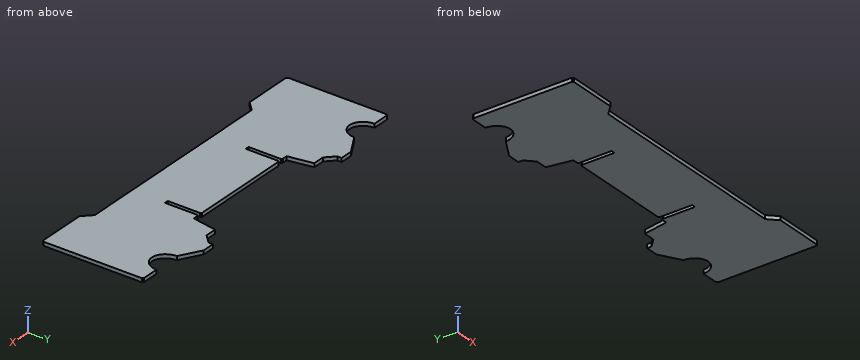
```python
from build123d import *

# Parameters (mm, degrees)
BOSS_EXTRUDE1_DEPTH = 3
SKETCH2_W           = 3
SKETCH2_H           = 4.791544689
CUT_EXTRUDE1_DEPTH  = 15
CHAMFER1_SIZE       = 1
CHAMFER2_SIZE       = 1


with BuildPart() as part:
    # Sketch1 → Boss-Extrude1 (new body)
    with BuildSketch(Plane.XY):
        with BuildLine():
            Line((93.184787819, -119.514382091), (261.489822447, -119.514382091))
            Line((261.489822447, -119.514382091), (268.560890259, -126.585449903))
            Line((268.560890259, -126.585449903), (308.560890259, -126.585449903))
            Line((308.560890259, -126.585449903), (308.560890259, -45.93363109))
            Line((308.560890259, -45.93363109), (294.267338786, -45.93363109))
            add(Edge.make_bspline(
                [(272.407878144, -45.934404782), (272.465337406, -47.438364471), (273.073186229, -50.465203155), (275.397677042, -54.367125899), (278.960411882, -57.115608226), (283.338040094, -58.12903526), (287.715596557, -57.115298346), (291.278136829, -54.366563828), (293.602351427, -50.464476548), (294.209985986, -47.437594843), (294.267338786, -45.93363109)],
                knots=[-1.525660034, -1.525660034, -1.525660034, -1.525660034, -1.144245025, -0.762830017, -0.381415008, 0, 0.381415008, 0.762830017, 1.144245025, 1.525660034, 1.525660034, 1.525660034, 1.525660034], degree=3))
            Line((272.407878144, -45.934404782), (256.337305133, -36.585449903))
            Line((256.337305133, -36.585449903), (246.337305133, -36.585449903))
            Line((246.337305133, -36.585449903), (246.337305133, -39.999663466))
            Line((246.337305133, -39.999663466), (239.751518696, -46.585449903))
            Line((239.751518696, -46.585449903), (230.574035326, -46.585449903))
            Line((230.574035326, -46.585449903), (227.127859803, -66.129682494))
            Line((227.127859803, -66.129682494), (127.546750463, -66.129682494))
            Line((127.546750463, -66.129682494), (124.10057494, -46.585449903))
            Line((124.10057494, -46.585449903), (114.923091571, -46.585449903))
            Line((114.923091571, -46.585449903), (108.337305133, -39.999663466))
            Line((108.337305133, -39.999663466), (108.337305133, -36.585449903))
            Line((108.337305133, -36.585449903), (98.337305133, -36.585449903))
            Line((98.337305133, -36.585449903), (82.267030577, -45.934761617))
            add(Edge.make_bspline(
                [(60.407579689, -45.934761617), (60.464998848, -47.438718586), (61.072758356, -50.465565598), (63.397111959, -54.367547882), (66.959733327, -57.116142381), (71.337305133, -58.129720884), (75.714876939, -57.116142381), (79.277498308, -54.367547882), (81.60185191, -50.465565598), (82.209611419, -47.438718586), (82.267030577, -45.934761617)],
                knots=[1.615943427, 1.615943427, 1.615943427, 1.615943427, 1.997355734, 2.37876804, 2.760180347, 3.141592654, 3.52300496, 3.904417267, 4.285829573, 4.66724188, 4.66724188, 4.66724188, 4.66724188], degree=3))
            Line((60.407579689, -45.934761617), (46.113720007, -45.934761617))
            Line((46.113720007, -45.934761617), (46.113720007, -126.585449903))
            Line((46.113720007, -126.585449903), (86.113720007, -126.585449903))
            Line((86.113720007, -126.585449903), (93.184787819, -119.514382091))
        make_face()
    extrude(amount=BOSS_EXTRUDE1_DEPTH)

    # Sketch2 → Cut-Extrude1 (cut)
    with BuildSketch(Plane(origin=(0, 0, 0), x_dir=(-1, 0, 0), z_dir=(0, 0, -1))):
        Polygon((-222.127859803, -66.129682494), (-222.127859803, -71.338137805), (-222.127859803, -92.822032293), (-219.127859803, -92.822032293), (-219.127859803, -71.338137805), (-219.127859803, -66.129682494), align=None)
        with Locations((-220.627859803, -63.73391015)):
            Rectangle(SKETCH2_W, SKETCH2_H)
        with Locations((-134.046750463, -63.73391015)):
            Rectangle(SKETCH2_W, SKETCH2_H)
        Polygon((-132.546750463, -66.129682494), (-135.546750463, -66.129682494), (-135.546750463, -71.338137805), (-135.546750463, -92.822032293), (-132.546750463, -92.822032293), (-132.546750463, -71.338137805), align=None)
    extrude(amount=-CUT_EXTRUDE1_DEPTH, mode=Mode.SUBTRACT)

    # Chamfer1
    chamfer1_edges = [part.edges().sort_by_distance(p)[0] for p in [
        (222.127859803, -66.129682494, 1.5),
        (219.127859803, -66.129682494, 1.5),
        (132.546750463, -66.129682494, 1.5),
        (135.546750463, -66.129682494, 1.5),
    ]]
    chamfer(chamfer1_edges, length=CHAMFER1_SIZE)

    # Chamfer2
    chamfer2_edges = [part.edges().sort_by_distance(p)[0] for p in [
        (308.560890259, -45.93363109, 1.5),
        (308.560890259, -126.585449903, 1.5),
        (46.113720007, -126.585449903, 1.5),
        (46.113720007, -45.934761617, 1.5),
    ]]
    chamfer(chamfer2_edges, length=CHAMFER2_SIZE)


solid = part.part
```
The model under review builds one solid part; all positions refer to its coordinate system, in mm. Round coordinates to 2 decimals unless told otherwise and drop trailing zeros. Write each loop counter-clockwise with the first axis right and the second up, starting at its lowest first coordinate (ties: lowest second). Pieces come first, ordered by that corner, then holes.
(1) Insertion check: pin 1 (1.5 mm diameter, centred on x = 201, z = 1.5, fed in from +Y); pin 2 (0.9 mm diameter, centred on x = 204.5, z = 1.5, fed in from -Y); pin 3 (1.5 mm diameter, centred on x = 117.5, z = 2, fed in from +Y). Each pin has a flat end and moves straight along its axis. Give the tip position at first contact, or say it passes through.
(2) We need section A-A on y = -85. Give the boundary of the cut face in (x, z), and give its area (3 significant figures).
(3) Wall thickness on L1, parallel to X at y = -88, z = 1.3; L2, parallel to X at y = -53.5, z = 2.05; L3, parallel to Y at x = 194, z = 0.75: over which ranges is each line inside the solid? List them lowest first.
(4) We need section B-B on x = 203.5. Give the boundary of the cut face in (y, z), and give its area (3 significant figures).
Findings below:
1. pin 1: stops at y = -66.13
1. pin 2: stops at y = -119.51
1. pin 3: stops at y = -46.59
2. outline: (46.11, 0) - (132.55, 0) - (132.55, 3) - (46.11, 3) - close; (135.55, 0) - (219.13, 0) - (219.13, 3) - (135.55, 3) - close; (222.13, 0) - (308.56, 0) - (308.56, 3) - (222.13, 3) - close
2. area: 769 mm2
3. L1: x = 46.11 to 132.55, 135.55 to 219.13, 222.13 to 308.56
3. L2: x = 46.11 to 63.05, 79.63 to 125.32, 229.35 to 275.05, 291.63 to 308.56
3. L3: y = -119.51 to -66.13
4. outline: (-119.51, 0) - (-66.13, 0) - (-66.13, 3) - (-119.51, 3) - close
4. area: 160 mm2
